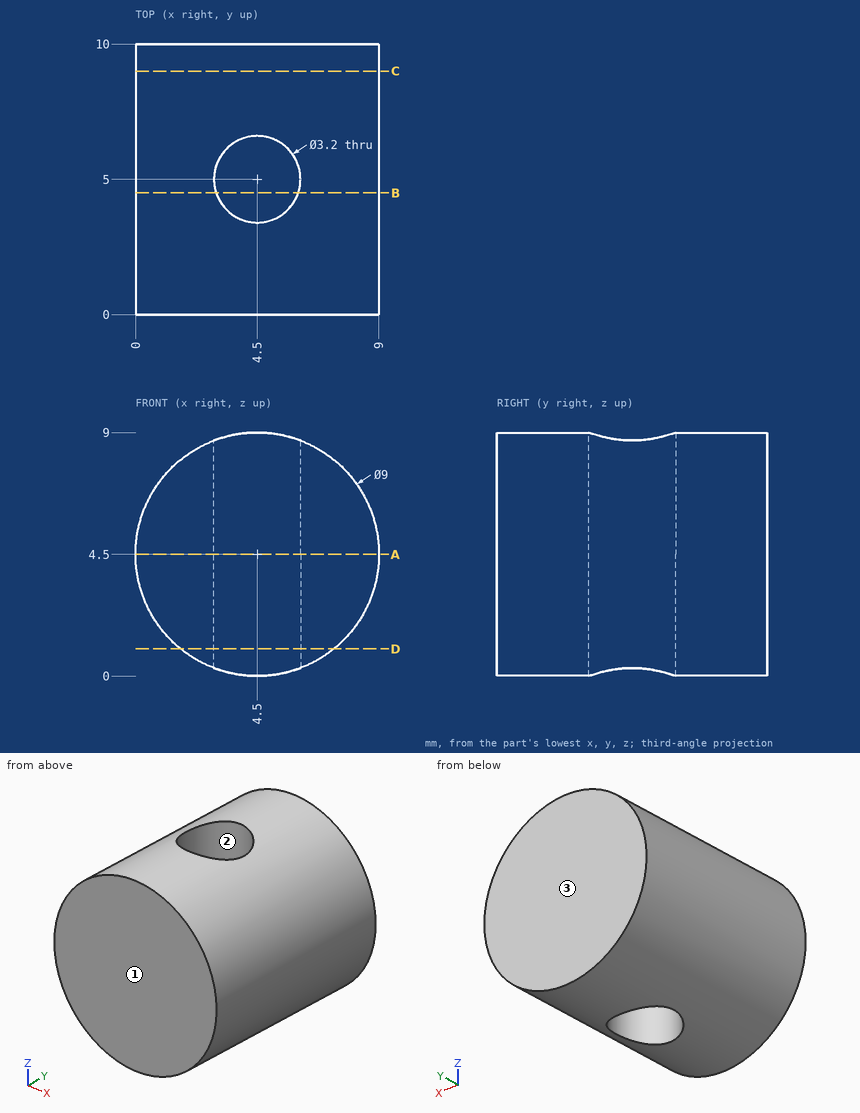
Here's the drawing with two shaded views (mm, measured from the low corner). I have some questions. Give positions to 0.01 mm unless a question says otherwise; leave off trailing zeros. Write each loop counter-clockwise with the first axis right and the second up, starting at its lowest first coordinate (ties: lowest second). Pieces come first, ordered by that corner, then holes. Notation, with made-up numbers: (86, 74.25) -> (114, 74.25) arc R25 cw to (114, 106.25) -> close; hole circle Ø4 at (55.25, 27). An arc over 180 degrees is marked (long way). Use one line per item in the form item = value.
1) If I drill on L1, parallel to Y at x = 4.5, z = 3; L2, parallel to X at y = 5, z = 5; L3, parallel to X at y = 6.25, z = 2.5, over which ranges is the centre line in solid material (lowest first)? Write a range as [from, to].
Verdict:
L1 = [0, 3.4], [6.6, 10]
L2 = [0.03, 2.9], [6.1, 8.97]
L3 = [0.47, 3.5], [5.5, 8.53]
2) Suppose I cut it at A-A (z = 4.5). Please give me the cut outline in (x, y), and give its area (3 significant figures).
Verdict:
outline = (0, 0) -> (9, 0) -> (9, 10) -> (0, 10) -> close; hole circle Ø3.2 at (4.5, 5)
area = 82.0 mm2
3) We'd pull the mould along Y, two halves only. Please class the marked faces 1, 2 and 3: +Y half, -Y half, draft (parallel to the pull), parting line (faces both ways), or undercut.
Verdict:
face_1 = -Y half
face_2 = undercut
face_3 = +Y half
4) Suppose I cut it at B-B (y = 4.5). Please give me the cut outline in (x, z), and give its area (3 significant figures).
Verdict:
outline = (2.98, 0.26) -> (2.98, 8.74) arc R4.5 ccw to start; (6.02, 0.26) arc R4.5 ccw to (6.02, 8.74) -> close
area = 36.8 mm2
5) Suppose I cut it at C-C (y = 9). Please give me the cut outline in (x, z), and give its area (3 significant figures).
Verdict:
outline = circle Ø9 at (4.5, 4.5)
area = 63.6 mm2
6) Suppose I cut it at D-D (z = 1). Please give me the cut outline in (x, y).
Verdict:
outline = (1.67, 0) -> (7.33, 0) -> (7.33, 10) -> (1.67, 10) -> close; hole circle Ø3.2 at (4.5, 5)
7) I'm going to push flat-ended pins straight in: pin 1 (5 mm diameter, centred on y = 1, z = 7.5, fed in from -X); pin 2 (3 mm diameter, centred on x = 6.5, y = 7.5, fed in from -Z); pin 3 (1 mm diameter, centred on x = 3, y = 4, fed in from -Z). Where does each tip first touch, or does it pass through?
Verdict:
pin_1 = 0.03
pin_2 = 0.03
pin_3 = 0.12
